```python
from build123d import *

# Parameters (mm, degrees)
F1_DEPTH      = 38.1
F2_T1_DEPTH   = 64.2282991577
F2_T3_DEPTH   = 53.4259096179
F2_T8_DEPTH   = 69.8505852304
F2_T13_DEPTH  = 69.8505852304
F2_T18_DEPTH  = 57.18488627
F2_T23_DEPTH  = 57.18488627
F2_T29_DEPTH  = 57.18488627
F2_T33_DEPTH  = 56.7864356516
F2_T40_DEPTH  = 56.7864356516
F2_T44_DEPTH  = 57.18488627
F3_R          = 5.5188922036
F4_R          = 5.08
F5_SIZE       = 5.08
F6_SIZE       = 5.08
F8_DEPTH      = 5.842
F8_DEPTH_BACK = 25.4


# Not quite as in the source:
# - a fillet or chamfer that OpenCascade refuses, or shapes differently, is made with other operations: its cross-section is extruded or revolved along the edge and cut away or added


with BuildPart() as f1:
    # F0 (on Front) → F1 (new body)
    with BuildSketch(Plane.XZ):
        Polygon((68.3197870099, -30.5711814668), (90.9013386944, -32.4848717284), (90.9013386944, -19.5518693537), (90.9013386944, -0.0529484335), (93.0701802755, 0), (60.7909710004, 0), (39.9160396704, 0), (35.1392942637, 5.0951969111), (26.685241969, 19.2868879506), (6.6764656577, 19.2868879506), (-19.6780025163, 19.2868879506), (-34.6921224135, 19.2868879506), (-59.0340113345, 0), (-76.2522614858, 0), (-85.7398739654, 0), (-102.7562974073, 0), (-102.7562974073, -29.6926991102), (-93.4295707114, -20.2366987188), (-86.7940447176, -20.2366987188), (-78.7120151127, -20.2366987188), (-76.6338963938, -20.2366987188), (-64.6562974073, -29.6926991102), (-40.7615778127, -29.6926991102), (-19.6780025163, -29.6926991102), (0, -29.6926991102), (14.0557177055, -29.6926991102), (30.2197870099, -29.6926991102), (39.1803090661, -19.5023065498), (56.2228657745, -19.5023065498), align=None)
    extrude(amount=F1_DEPTH)

    # F2: chamfer of 5.08 on 6 edges, made by hand

    # F2_s2 → F2_t1 (cut)
    with BuildSketch(Plane.XZ.offset(-13.0641495789)):
        Polygon((-102.7562974073, -5.08), (-97.6762974073, 0), (-102.7562974073, 0), align=None)
    extrude(amount=F2_T1_DEPTH, mode=Mode.SUBTRACT)

    # F2_s4 → F2_t3 (cut)
    with BuildSketch(Plane.XZ.offset(-7.6629548089)):
        Polygon((23.7983706465, 19.2868879506), (28.1626838525, 16.8067283763), (26.685241969, 19.2868879506), align=None)
    extrude(amount=F2_T3_DEPTH, mode=Mode.SUBTRACT)


with BuildPart() as f2_tool6:
    # F2_s7 → F2_t8 (new body)
    with BuildSketch(Plane.YZ.offset(-115.8204469861)):
        Polygon((-38.1, -5.08), (-33.02, 0), (-38.1, 0), align=None)
    extrude(amount=F2_T8_DEPTH)

    split(bisect_by=Plane(origin=(-22.7676995967, 0, 28.7350046307), x_dir=(0, 1, 0), z_dir=(-0.6210240643, 0, 0.7837914975)), keep=Keep.TOP)


with BuildPart() as f1_1:
    add(f1.part)

    # F2_t5: cut F2_tool6
    add(f2_tool6.part, mode=Mode.SUBTRACT)


with BuildPart() as f2_tool11:
    # F2_s12 → F2_t13 (new body)
    with BuildSketch(Plane.YZ.offset(-45.9698617557)):
        Polygon((-5.08, 0), (0, -5.08), (0, 0), align=None)
    extrude(amount=-F2_T13_DEPTH)

    split(bisect_by=Plane(origin=(-22.7676995967, 0, 28.7350046307), x_dir=(0, 1, 0), z_dir=(-0.6210240643, 0, 0.7837914975)), keep=Keep.TOP)


with BuildPart() as f1_2:
    add(f1_1.part)

    # F2_t10: cut F2_tool11
    add(f2_tool11.part, mode=Mode.SUBTRACT)


with BuildPart() as f2_tool16:
    # F2_s17 → F2_t18 (new body)
    with BuildSketch(Plane(origin=(-1.6848534543, 0, -1.3349654126), x_dir=(0, 1, 0), z_dir=(-0.7837914975, 0, -0.6210240643))):
        Polygon((-38.1, -31.5815416486), (-33.02, -36.6615416486), (-38.1, -36.6615416486), align=None)
    extrude(amount=F2_T18_DEPTH)

    split(bisect_by=Plane.XY, keep=Keep.TOP)


with BuildPart() as f1_3:
    add(f1_2.part)

    # F2_t15: cut F2_tool16
    add(f2_tool16.part, mode=Mode.SUBTRACT)


with BuildPart() as f2_tool21:
    # F2_s22 → F2_t23 (new body)
    with BuildSketch(Plane(origin=(-1.6848534543, 0, -1.3349654126), x_dir=(0, 1, 0), z_dir=(-0.7837914975, 0, -0.6210240643))):
        Polygon((-5.08, -36.6615416486), (0, -31.5815416486), (0, -36.6615416486), align=None)
    extrude(amount=F2_T23_DEPTH)

    split(bisect_by=Plane.XY, keep=Keep.TOP)


with BuildPart() as f1_4:
    add(f1_3.part)

    # F2_t20: cut F2_tool21
    add(f2_tool21.part, mode=Mode.SUBTRACT)


with BuildPart() as f2_tool27:
    # F2_s28 → F2_t29 (new body)
    with BuildSketch(Plane(origin=(-1.6848534543, 0, -1.3349654126), x_dir=(0, 1, 0), z_dir=(-0.7837914975, 0, -0.6210240643))):
        Polygon((-38.1, -31.5815416486), (-33.02, -36.6615416486), (-38.1, -36.6615416486), align=None)
    extrude(amount=F2_T29_DEPTH)

    split(bisect_by=Plane.XY, keep=Keep.BOTTOM)


with BuildPart() as f2_tool31:
    # F2_s32 → F2_t33 (new body)
    with BuildSketch(Plane.YZ.offset(-102.7562974073)):
        Polygon((-38.1, -5.08), (-33.02, 0), (-38.1, 0), align=None)
    extrude(amount=F2_T33_DEPTH)

    split(bisect_by=Plane(origin=(-22.7676995967, 0, 28.7350046307), x_dir=(0, 1, 0), z_dir=(0.6210240643, 0, -0.7837914975)), keep=Keep.TOP)


with BuildPart() as f2_tool27_1:
    add(f2_tool27.part)

    # F2_t35: intersect F2_tool31
    add(f2_tool31.part, mode=Mode.INTERSECT)


with BuildPart() as f1_5:
    add(f1_4.part)

    # F2_t25: cut F2_tool27
    add(f2_tool27_1.part, mode=Mode.SUBTRACT)


with BuildPart() as f2_tool38:
    # F2_s39 → F2_t40 (new body)
    with BuildSketch(Plane.YZ.offset(-45.9698617557)):
        Polygon((-5.08, 0), (0, -5.08), (0, 0), align=None)
    extrude(amount=-F2_T40_DEPTH)

    split(bisect_by=Plane(origin=(-22.7676995967, 0, 28.7350046307), x_dir=(0, 1, 0), z_dir=(0.6210240643, 0, -0.7837914975)), keep=Keep.TOP)


with BuildPart() as f2_tool42:
    # F2_s43 → F2_t44 (new body)
    with BuildSketch(Plane(origin=(-1.6848534543, 0, -1.3349654126), x_dir=(0, 1, 0), z_dir=(-0.7837914975, 0, -0.6210240643))):
        Polygon((-5.08, -36.6615416486), (0, -31.5815416486), (0, -36.6615416486), align=None)
    extrude(amount=F2_T44_DEPTH)

    split(bisect_by=Plane.XY, keep=Keep.BOTTOM)


with BuildPart() as f2_tool38_1:
    add(f2_tool38.part)

    # F2_t46: intersect F2_tool42
    add(f2_tool42.part, mode=Mode.INTERSECT)


with BuildPart() as f1_6:
    add(f1_5.part)

    # F2_t36: cut F2_tool38
    add(f2_tool38_1.part, mode=Mode.SUBTRACT)

    # F3
    f3_edges = [f1_6.edges().sort_by_distance(p)[0] for p in [
        (62.271326, 0, -25.036744),
        (47.701587, 0, -19.502307),
        (34.700048, 0, -24.597503),
    ]]
    fillet(f3_edges, radius=F3_R)

    # F4
    f4_edges = [f1_6.edges().sort_by_distance(p)[0] for p in [
        (34.700048, -38.1, -24.597503),
        (47.701587, -38.1, -19.502307),
        (62.271326, -38.1, -25.036744),
        (-70.645097, 0, -24.964699),
        (-85.031734, 0, -20.236699),
        (-98.092934, 0, -24.964699),
        (-85.031734, -38.1, -20.236699),
        (-70.645097, -38.1, -24.964699),
        (-98.092934, -38.1, -24.964699),
    ]]
    fillet(f4_edges, radius=F4_R)

    # F5
    f5_edges = [f1_6.edges().sort_by_distance(p)[0] for p in [
        (66.49311, -38.1, 0),
        (66.49311, 0, 0),
    ]]
    chamfer(f5_edges, length=F5_SIZE)

    # F6
    f6_edges = [f1_6.edges().sort_by_distance(p)[0] for p in [
        (-1.356857, 0, 19.286888),
        (-1.356857, -38.1, 19.286888),
    ]]
    chamfer(f6_edges, length=F6_SIZE)

    # F7 (on face) → F8 (join, two sides)
    with BuildSketch(Plane(origin=(0, 0, -29.6926991102), x_dir=(1, 0, 0), z_dir=(0, 0, -1))) as f8_sk:
        Polygon((-102.5345399976, 24.3232287467), (-102.5345399976, 12.4534405768), (90.11746943, 12.4534405768), (91.410189867, 12.4534405768), (91.410189867, 24.3232287467), align=None)
    extrude(amount=F8_DEPTH)
    extrude(f8_sk.sketch, amount=-F8_DEPTH_BACK)


solid = f1_6.part
```
The listing builds one solid part. Answer for the finished solid, in the listing's coordinates (mm). A direction names the side the tool comes from. Round coordinates to 2 decimals unless told otherwise and drop trailing zeros. Loops run counter-clockwise (first coordinate to the right, second up) from the corner with the lowest first, then second, coordinate; pieces in that order, holes last.
1) A cutting plane is placed at D-D on y = -27.5. Determine the outline of the cut face in (x, z), plus the area to 3 significant figures.
Outcome:
outline: (-102.76, -29.69) - (-93.43, -20.24) - (-76.63, -20.24) - (-64.66, -29.69) - (30.22, -29.69) - (39.18, -19.5) - (56.22, -19.5) - (68.32, -30.57) - (90.9, -32.48) - (90.9, -0.05) - (93.07, 0) - (39.92, 0) - (35.14, 5.1) - (28.16, 16.81) - (23.8, 19.29) - (-34.69, 19.29) - (-59.03, 0) - (-97.68, 0) - (-102.76, -5.08) - close
area: 6,770 mm2
2) Consider line 1 (X direction, y = -3, z = -24); line 2 (X direction, y = -5, z = -27); line 3 (Z direction, x = -12, y = -9.5). Determine where each line is inside the solid, lowest interval first.
Outcome:
line 1: x = -102.76 to -97.77, -71.15 to 34.42, 62.04 to 90.9
line 2: x = -102.76 to -100.1, -68.07 to 32.55, 64.45 to 90.9
line 3: z = -29.69 to 19.29
3) A cutting plane is placed at C-C on z = 2. Determine the outline of the cut face in (x, y).
Outcome:
outline: (-56.51, -33.02) - (-48.33, -38.1) - (38.04, -38.1) - (38.04, 0) - (-48.33, 0) - (-56.51, -5.08) - close
4) For faces 1 (the face through (-78, -19, 0)), 2 (the face through (-85.07, -36.65, -18.71)), 3 (the face through (48, -9, -19.502)), determine the directions among +Z, -Z, +X, -X, +Y, -Y from which every point of the face is accessible in a straight line to the end or side of a thin tool.
Outcome:
face 1: +Z, -X, +Y, -Y
face 2: -Z, -Y
face 3: -Z, +Y
5) Given P1, Ø6, axis at x = -82.5, y = -7.5, coming from the -Z side; P2, Ø2, axis at x = 46, y = -9, coming from the -Z side; P3, Ø0.6, axis at y = -16.5, z = -4.5, coming from the -X side, each flat-ended and moving along its own axis, determine where each tip first touches the part or whether it passes through.
Outcome:
P1: stops at z = -20.24
P2: stops at z = -19.5
P3: stops at x = -102.53
6) For a pull along X with two mould halves and no side action, classify faces 4 (the face through (-7, -38.1, -9)), 5 (the face through (79.452, -31.115, -31.515)), 6 (the face through (34.637, -28.611, -24.669)), 7 (the face through (-98.36, -36.65, -23.06)) as released by +X, released by -X, zero draft, split by the parting line, or undercut.
Outcome:
face 4: zero draft
face 5: released by -X
face 6: undercut
face 7: undercut
7) A cutting plane is placed at B-B on x = -29. Determine the outline of the cut face in (y, z).
Outcome:
outline: (-38.1, -29.69) - (-24.32, -29.69) - (-24.32, -35.53) - (-12.45, -35.53) - (-12.45, -29.69) - (0, -29.69) - (0, 14.21) - (-5.08, 19.29) - (-33.02, 19.29) - (-38.1, 14.21) - close
8) A cutting plane is placed at A-A on y = -18.5. Determine the outline of the cut face in (x, z), plus the area to 3 significant figures.
Outcome:
outline: (-102.76, -29.69) - (-102.53, -29.47) - (-102.53, -35.53) - (91.41, -35.53) - (91.41, -4.29) - (90.9, -4.29) - (90.9, -0.05) - (93.07, 0) - (39.92, 0) - (35.14, 5.1) - (28.16, 16.81) - (23.8, 19.29) - (-34.69, 19.29) - (-59.03, 0) - (-97.68, 0) - (-101.97, -4.29) - (-102.53, -4.29) - (-102.53, -4.86) - (-102.76, -5.08) - close
area: 8,410 mm2
